Geometry: final body of the model. Coordinates: model frame, mm. Face numbers are marked on the shaded views. A direction names the side the tool comes from. Give positions to 0.01 mm unless a question says otherwise; leave off trailing zeros. Write each loop counter-clockwise with the first axis right and the second up, starting at its lowest first coordinate (ties: lowest second). Pieces come first, ordered by that corner, then holes.
Q1. Section A-A (y = 1.25). Return the cut outline in (x, z).
Q2. Reachability of the marked faces 4, 5, 6, 7 and 8 from +Z, -Z, +X, -X, +Y, -Y: full face, straight path, thin tool, end or side. Return the list, or none.
Q3. Section D-D (y = 13.5). Return the cut outline in (x, z).
Q4. Line query: line 1 (X direction, y = -2.5, z = 10); line 2 (X direction, y = 15.25, z = 10); line 3 (Y direction, x = 8.6, z = 8). Output: solid intervals per line, ascending.
Q5. Pin query (flat end, axial travel): pin 1 Ø8 at (y, z) = (13, 15) entering from -X; pin 2 Ø1 at (x, z) = (7.5, 16) entering from -Y; pin 3 Ø6 at (x, y) = (-5.5, -6) entering from +Z; pin 4 Ø5 at (x, y) = (7.5, 2.5) entering from +Z. Return the tip coordinate at first contact, or that it passes through.
Q6. Section C-C (x = 18.5). Return the cut outline in (y, z).
Q7. Section B-B (z = 16.75). Return the cut outline in (x, y), plus the area to 3 significant figures.
Q8. Mould query, pull axis X, two halves, no side actions, for the marked faces 1, 2 and 3. Classes: +X half, -X half, draft (parallel to the pull), parting line (faces both ways), or undercut.
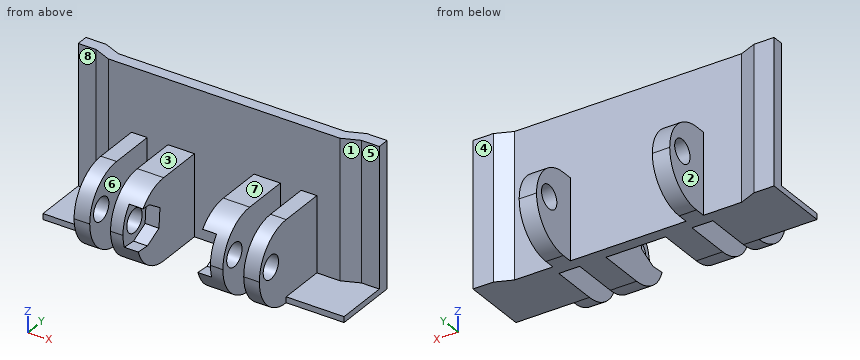
from build123d import *

# Parameters (mm, degrees)
SKETCH2_W                 = 5
SKETCH2_H                 = 15
BOSS_EXTRUDE1_DEPTH       = 14
BOSS_EXTRUDE1_2_DEPTH     = 14
BOSS_EXTRUDE3_DEPTH       = 25
SKETCH5_W                 = 3
SKETCH5_H                 = 8.8
BOSS_EXTRUDE4_DEPTH       = 14
SKETCH7_W                 = 3
SKETCH7_H                 = 15
BOSS_EXTRUDE5_DEPTH       = 14
SKETCH15_W                = 0.3
SKETCH15_H                = 14
CUT_EXTRUDE2_DEPTH        = 15
SKETCH16_W                = 0.15
SKETCH16_H                = 14
CUT_EXTRUDE3_DEPTH        = 15
FILLET1_R                 = 7
F_4_0MM_DOWEL_HOLE2_D     = 4
FILLET2_R                 = 7
F_4_0MM_DOWEL_HOLE1_D     = 4
F_4_0MM_DOWEL_HOLE1_DEPTH = 26
F_4_0MM_DOWEL_HOLE1_TIP   = 1.201721238
BOSS_EXTRUDE6_DEPTH       = 1
CUT_EXTRUDE4_DEPTH        = 2.4


with BuildPart() as part:
    # Sketch2 → Boss-Extrude1 (new body)
    with BuildSketch(Plane.XY):
        with Locations((-7.5, -1.5)):
            Rectangle(SKETCH2_W, SKETCH2_H)
    extrude(amount=BOSS_EXTRUDE1_DEPTH)



with BuildPart() as body_2:
    # Sketch2 → Boss-Extrude1 2 (new body)
    with BuildSketch(Plane.XY):
        with Locations((7.5, -1.5)):
            Rectangle(SKETCH2_W, SKETCH2_H)
    extrude(amount=BOSS_EXTRUDE1_2_DEPTH)


with BuildPart() as part_1:
    add(part.part)

    add(body_2.part)  # Boss-Extrude3 merges body 2
    # Sketch4 → Boss-Extrude3 (add)
    with BuildSketch(Plane.XY):
        Polygon((-10, 6), (-20, 6), (-22.901603942, 7.206366686), (-26, 7.206366686), (-26, 9.206366686), (-22.502408858, 9.206366686), (-19.600804916, 8), (-10, 8), (10, 8), (19.600804916, 8), (22.502408858, 9.206366686), (26, 9.206366686), (26, 7.206366686), (22.901603942, 7.206366686), (20, 6), (10, 6), align=None)
    extrude(amount=BOSS_EXTRUDE3_DEPTH)

    # Sketch5 → Boss-Extrude4 (add)
    with BuildSketch(Plane.XY):
        with Locations((-11.5, 12.4)):
            Rectangle(SKETCH5_W, SKETCH5_H)
        with Locations((11.5, 12.4)):
            Rectangle(SKETCH5_W, SKETCH5_H)
    extrude(amount=BOSS_EXTRUDE4_DEPTH)

    # Sketch7 → Boss-Extrude5 (add)
    with BuildSketch(Plane.XY):
        with Locations((-14.5, -1.5)):
            Rectangle(SKETCH7_W, SKETCH7_H)
        with Locations((14.5, -1.5)):
            Rectangle(SKETCH7_W, SKETCH7_H)
    extrude(amount=BOSS_EXTRUDE5_DEPTH)

    # Sketch15 → Cut-Extrude2 (cut)
    with BuildSketch(Plane.XZ.offset(9)):
        with Locations((-9.85, 7)):
            Rectangle(SKETCH15_W, SKETCH15_H)
        with Locations((9.85, 7)):
            Rectangle(SKETCH15_W, SKETCH15_H)
        with Locations((-13.15, 7)):
            Rectangle(SKETCH15_W, SKETCH15_H)
        with Locations((13.15, 7)):
            Rectangle(SKETCH15_W, SKETCH15_H)
    extrude(amount=-CUT_EXTRUDE2_DEPTH, mode=Mode.SUBTRACT)

    # Sketch16 → Cut-Extrude3 (cut)
    with BuildSketch(Plane.XZ.offset(9)):
        with Locations((-5.075, 7)):
            Rectangle(SKETCH16_W, SKETCH16_H)
        with Locations((5.075, 7)):
            Rectangle(SKETCH16_W, SKETCH16_H)
    extrude(amount=-CUT_EXTRUDE3_DEPTH, mode=Mode.SUBTRACT)

    # Fillet1
    fillet1_edges = [part_1.edges().sort_by_distance(p)[0] for p in [
        (7.425, -9, 0),
        (7.425, -9, 14),
        (-7.425, -9, 0),
        (-7.425, -9, 14),
        (-14.65, -9, 0),
        (-14.65, -9, 14),
        (14.65, -9, 14),
        (14.65, -9, 0),
    ]]
    fillet(fillet1_edges, radius=FILLET1_R - 0.0001)  # a hair under: the kernel refuses the full size

    # Ø4.0mm Dowel Hole2 (through all)
    with Locations(Plane(origin=(16, 0, 0), x_dir=(0, 0, -1), z_dir=(1, 0, 0))):
        with Locations((-8, -6)):
            Hole(F_4_0MM_DOWEL_HOLE2_D / 2)

    # Fillet2
    fillet2_edges = [part_1.edges().sort_by_distance(p)[0] for p in [
        (-11.5, 16.8, 0),
        (-11.5, 16.8, 14),
        (11.5, 16.8, 0),
        (11.5, 16.8, 14),
    ]]
    fillet(fillet2_edges, radius=FILLET2_R - 0.0001)  # a hair under: the kernel refuses the full size

    # Ø4.0mm Dowel Hole1
    with Locations(Plane(origin=(13, 0, 0), x_dir=(0, 0, -1), z_dir=(1, 0, 0))):
        with Locations((-8, 13.5)):
            Hole(F_4_0MM_DOWEL_HOLE1_D / 2, depth=F_4_0MM_DOWEL_HOLE1_DEPTH)
            with Locations((0, 0, -(F_4_0MM_DOWEL_HOLE1_DEPTH + F_4_0MM_DOWEL_HOLE1_TIP / 2))):  # 118° drill point
                Cone(0, F_4_0MM_DOWEL_HOLE1_D / 2, F_4_0MM_DOWEL_HOLE1_TIP, mode=Mode.SUBTRACT)

    # Sketch14 → Boss-Extrude6 (add)
    with BuildSketch(Plane.XY):
        Polygon((-22.901603942, 7.206366686), (-26, 7.206366686), (-26, -2), (-16, -2), (-16, 6), (-20, 6), align=None)
        Polygon((20, 6), (16, 6), (16, -2), (26, -2), (26, 7.206366686), (22.901603942, 7.206366686), align=None)
    extrude(amount=BOSS_EXTRUDE6_DEPTH)

    # Sketch18 → Cut-Extrude4 (cut)
    with BuildSketch(Plane(origin=(-5.15, 0, 0), x_dir=(0, 0, -1), z_dir=(1, 0, 0))):
        Polygon((-6.110899152, -3.235107358), (-9.449916842, -2.981544355), (-11.33901769, -5.746436996), (-12.466071308, -20.587923763), (-5.788035927, -21.095049771), (-4.66098231, -6.253563004), align=None)
    cut_extrude4 = extrude(amount=-CUT_EXTRUDE4_DEPTH, mode=Mode.SUBTRACT)

    # Mirror1: Cut-Extrude4 across plane
    add(cut_extrude4.mirror(Plane(origin=(0, 0, 0), x_dir=(0, 0, 1), z_dir=(1, 0, 0))), mode=Mode.SUBTRACT)


solid = part_1.part
Computed:
1. outline: (-26, 0) - (-13.3, 0) - (-13.3, 14) - (-16, 14) - (-16, 1) - (-26, 1) - close; (-9.7, 0) - (-5.15, 0) - (-5.15, 14) - (-9.7, 14) - close; (5.15, 0) - (9.7, 0) - (9.7, 14) - (5.15, 14) - close; (13.3, 0) - (26, 0) - (26, 1) - (16, 1) - (16, 14) - (13.3, 14) - close
2. face 4: +Z, -Z, +X, +Y
2. face 5: +Z, +X, -Y
2. face 6: +Z, -Z, -Y
2. face 7: +Z, +X, -X, -Y
2. face 8: +Z, -X, -Y
3. outline: (-13, 1.06) - (-10, 1.06) - (-10, 6) - (-13, 6) - close; (-13, 10) - (-10, 10) - (-10, 12.94) - (-13, 12.94) - close; (10, 1.06) - (13, 1.06) - (13, 6) - (10, 6) - close; (10, 10) - (13, 10) - (13, 12.94) - (10, 12.94) - close
4. line 1: x = -16 to -13.3, -9.7 to -5.15, 5.15 to 9.7, 13.3 to 16
4. line 2: x = -13 to -10, 10 to 13
4. line 3: y = -8.93 to -8, -4 to 8
5. pin 1: stops at x = -26
5. pin 2: stops at y = 6
5. pin 3: stops at z = 13.93
5. pin 4: stops at z = 14
6. outline: (-2, 0) - (8, 0) - (8, 25) - (6, 25) - (6, 1) - (-2, 1) - close
7. outline: (-26, 7.21) - (-22.9, 7.21) - (-20, 6) - (20, 6) - (22.9, 7.21) - (26, 7.21) - (26, 9.21) - (22.5, 9.21) - (19.6, 8) - (-19.6, 8) - (-22.5, 9.21) - (-26, 9.21) - close
7. area: 105 mm2
8. face 1: +X half
8. face 2: undercut
8. face 3: draft
